Autodesk Inventor part; units mm, degrees
ref_plane "YZ Plane" through (0, 0, 0) normal (1, 0, 0) x (0, 1, 0)
ref_plane "XZ Plane" through (0, 0, 0) normal (0, 1, 0) x (-1, 0, 0)
ref_plane "XY Plane" through (0, 0, 0) normal (0, 0, 1) x (1, 0, 0)
sketch "Sketch1" plane through (0, 0, 0) normal (0, 0, 1) x (1, 0, 0)
  line L0 (-25, 37.5) -> (25, 37.5)
  line L1 (25, 37.5) -> (25, -37.5)
  line L2 (25, -37.5) -> (-25, -37.5)
  line L3 (-25, -37.5) -> (-25, 37.5)
  point P0 (0, 0)
  dimension "d0" = 50
  dimension "d1" = 75
  dimension "d2" = 37.5
  dimension "d3" = 25
extrude "Extrusion1" add sketch "Sketch1" along normal blind 10
sketch "Sketch2" plane through (0, 0, 10) normal (0, 0, 1) x (1, 0, 0)
  point P0 (0, 0)
  point P1 (20, -33.75)
  point P2 (-20, -33.75)
  point P3 (-20, 33.75)
  point P4 (20, 33.75)
  dimension "d6" = 40
  dimension "d7" = 20
  dimension "d8" = 67.5
  dimension "d9" = 33.75
hole "Hole1" at (20, -33.75, 10) at (-20, -33.75, 10) at (-20, 33.75, 10) at (20, 33.75, 10) direction (0, 0, -1) diameter 4.5 depth 9.525 tip angle 118
sketch "Sketch3" plane through (0, 0, 10) normal (0, 0, 1) x (1, 0, 0)
  line L0 (-17.5, -30) -> (17.5, -30)
  line L1 (17.5, -30) -> (17.5, 30)
  line L2 (17.5, 30) -> (-17.5, 30)
  line L3 (-17.5, 30) -> (-17.5, -30)
  line L4 (-12.5, -25) -> (12.5, -25)
  line L5 (12.5, -25) -> (12.5, 25)
  line L6 (12.5, 25) -> (-12.5, 25)
  line L7 (-12.5, 25) -> (-12.5, -25)
  point P0 (0, 0)
  dimension "d19" = 35
  dimension "d22" = 60
  dimension "d23" = 30
  dimension "d24" = 5
  dimension "d26" = 17.5
  dimension "d27" = 5
  dimension "d29" = 5
  dimension "d30" = 5
extrude "Extrusion2" cut sketch "Sketch3" against normal blind 6
equation "\"d27\" = d24"
equation "\"d29\" = d24"
equation "\"d30\" = d24"
properties part number "filipeSampleHolderBase"
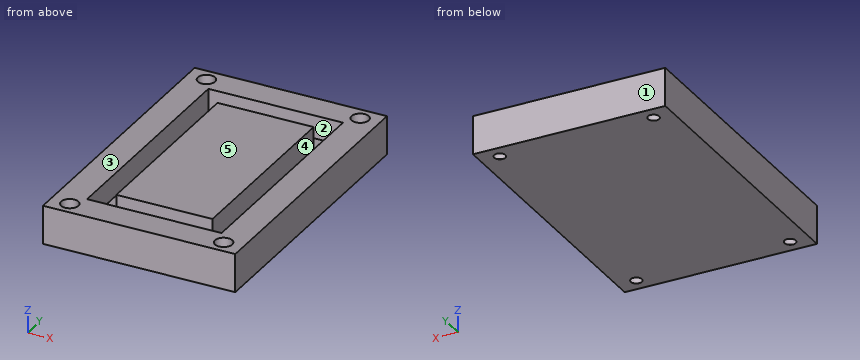
Could you check a few things on this model? Use its own coordinates, in mm. Face numbers are marked on the shaded views. A direction names the side the tool comes from. Coordinates: 2 decimals unless noted, no trailing zeros. Write each loop counter-clockwise with the first axis right and the second up, starting at its lowest first coordinate (ties: lowest second). Pieces come first, ordered by that corner, then holes. Notation, with made-up numbers: (52.5, 78) - (93.5, 78) arc R12 ccw to (93.5, 91) - close; hole circle Ø7 at (81, 64). An arc over 180 degrees is marked (long way). Write item = value, one per line.
1) Suppose I cut it at D-D on y = -33.75. Please give me the cut outline in (x, z) (3 decimals), plus the area to 3 significant figures.
Result set:
outline = (-25, 0) - (-21.459, 0) - (-22.25, 0.475) - (-22.25, 10) - (-25, 10) - close; (-18.541, 0) - (18.541, 0) - (17.75, 0.475) - (17.75, 10) - (-17.75, 10) - (-17.75, 0.475) - close; (21.459, 0) - (25, 0) - (25, 10) - (22.25, 10) - (22.25, 0.475) - close
area = 411 mm2
2) Suppose I cut it at C-C on x = -11. Please give me the cut outline in (y, z), plus the area to 3 significant figures.
Result set:
outline = (-37.5, 0) - (37.5, 0) - (37.5, 10) - (30, 10) - (30, 4) - (25, 4) - (25, 10) - (-25, 10) - (-25, 4) - (-30, 4) - (-30, 10) - (-37.5, 10) - close
area = 690 mm2
3) Suppose I cut it at B-B on y = -26. Please give me the cut outline in (x, z), plus the area to 3 significant figures.
Result set:
outline = (-25, 0) - (25, 0) - (25, 10) - (17.5, 10) - (17.5, 4) - (-17.5, 4) - (-17.5, 10) - (-25, 10) - close
area = 290 mm2
4) Suppose I cut it at A-A on z = 7.5. Please give me the cut outline in (x, y).
Result set:
outline = (-25, -37.5) - (25, -37.5) - (25, 37.5) - (-25, 37.5) - close; (-12.5, -25) - (12.5, -25) - (12.5, 25) - (-12.5, 25) - close; hole circle Ø4.5 at (-20, -33.75); hole circle Ø4.5 at (-20, 33.75); hole (-17.5, -30) - (17.5, -30) - (17.5, 30) - (-17.5, 30) - close; hole circle Ø4.5 at (20, -33.75); hole circle Ø4.5 at (20, 33.75)
5) Please list where these lines run through material, in increasing order: line 1 (X direction, y = -3.5, z = 6.5); line 2 (Y direction, x = -6, z = 6.25); line 3 (X direction, y = 33.75, z = 7.75). Write a range as [from, to].
Result set:
line_1 = [-25, -17.5], [-12.5, 12.5], [17.5, 25]
line_2 = [-37.5, -30], [-25, 25], [30, 37.5]
line_3 = [-25, -22.25], [-17.75, 17.75], [22.25, 25]
6) We'd pull the mould along Y, two halves only. Please class the marked faces 1, 2 and 3: +Y half, -Y half, draft (parallel to the pull), parting line (faces both ways), or undercut.
Result set:
face_1 = +Y half
face_2 = undercut
face_3 = draft
7) Will this pin go through, and if not, where does the flat tip stop? pin 1 Ø3 at (x, y) = (-15.5, -26) entering from +Z.
Result set:
pin_1 = 4
8) For the marked faces 4 and 5, which set-ups out of +Z, -Z, +X, -X, +Y, -Y let a thin tool reach every point of the face, with its end or its side?
Result set:
face_4 = +Z
face_5 = +Z, +X, -X, +Y, -Y
